The listing builds one solid part. Answer for the finished solid, in the listing's coordinates (mm). Face numbers are marked on the shaded views. A direction names the side the tool comes from. Coordinates: 2 decimals unless noted, no trailing zeros. Loops run counter-clockwise (first coordinate to the right, second up) from the corner with the lowest first, then second, coordinate; pieces in that order, holes last. Notation, with made-up numbers: M 55.5,58 L 91.5,58 A20 ccw 91.5,82 Z; hole C -5,-32 d1. An arc over 180 degrees is marked long. Answer as a JSON object with one key per item and string values. Group by question number.
1. A cutting plane is placed at B-B on x = 25.5. Give the vertices of the cut face in (y, z).
2. A cutting plane is placed at A-A on z = 12. Give the vertices of the cut face in (x, y) (3 decimals).
3. A cutting plane is placed at C-C on x = 12. Give the vertices of the cut face in (y, z), and give its area (3 significant figures).
4. Given pin 1 (4 mm diameter, centred on x = 14, z = 34, fed in from -Y); pin 2 (6 mm diameter, centred on x = -16.5, y = 81.5, fed in from -Z), each flat-ended and moving along its own axis, determine where each tip first touches the part or whether it passes through.
5. Determine the mould class of the marked faces 3, 4, 5 and 6 for opening direction X: released by +X, released by -X, zero draft, split by the parting line, or undercut.
6. For the marked faces 1 and 2, determine the directions among +Z, -Z, +X, -X, +Y, -Y from which every point of the face is accessible in a straight line to the end or side of a thin tool.
7. Straight lines are drawn through the part: L1, parallel to X at y = 76, z = 23.5; L2, parallel to Y at x = -11, z = 30; L3, parallel to Y at x = 19.5, z = 17.5. For each, find the intervals that lie inside material, in ascending order.
from build123d import *

# Parameters (mm, degrees)
BOSS_EXTRUDE1_DEPTH = 50.8
FILLET1_R           = 2.54


with BuildPart() as part:
    # Sketch1 → Boss-Extrude1 (new body)
    with BuildSketch(Plane.XY):
        with BuildLine():
            Line((-12.7, 73.846320157), (12.7, 73.846320157))
            Line((12.7, 73.846320157), (15.605843118, 90.742841512))
            ThreePointArc((15.605843118, 90.742841512), (23.776020133, 88.952270863), (31.75, 86.427675689))
            Line((31.75, 86.427675689), (31.75, 99.102275689))
            Line((31.75, 99.102275689), (-31.75, 99.102275689))
            Line((-31.75, 99.102275689), (-31.75, 86.427675689))
            ThreePointArc((-31.75, 86.427675689), (-23.776020133, 88.952270863), (-15.605843118, 90.742841512))
            Line((-15.605843118, 90.742841512), (-12.7, 73.846320157))
        make_face()
    extrude(amount=BOSS_EXTRUDE1_DEPTH)

    # Fillet1
    fillet1_edges = [part.edges().sort_by_distance(p)[0] for p in [
        (12.7, 73.846320157, 25.4),
        (-12.7, 73.846320157, 25.4),
        (-15.605843118, 90.742841512, 25.4),
        (15.605843118, 90.742841512, 25.4),
    ]]
    fillet(fillet1_edges, radius=FILLET1_R)


solid = part.part
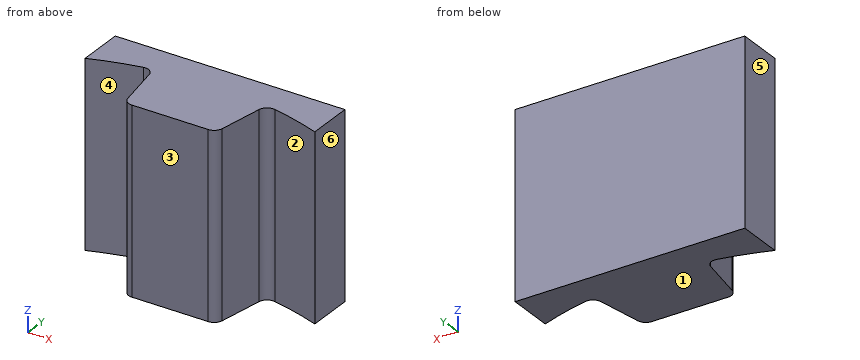
From the geometry:
{
 "1": {"outline": "M 88.47,0 L 99.1,0 L 99.1,50.8 L 88.47,50.8 Z"},
 "2": {"outline": "M -31.75,86.428 A92.075 cw -18.174,90.264 A2.54 cw -15.169,88.204 L -13.063,75.956 A2.54 ccw -10.56,73.846 L 10.56,73.846 A2.54 ccw 13.063,75.956 L 15.169,88.204 A2.54 cw 18.174,90.264 A92.075 cw 31.75,86.428 L 31.75,99.102 L -31.75,99.102 Z"},
 "3": {"outline": "M 74.29,0 L 99.1,0 L 99.1,50.8 L 74.29,50.8 Z", "area": "1,260 mm²"},
 "4": {"pin 1": "stops at y = 74.29", "pin 2": "stops at z = 0"},
 "5": {"face 3": "zero draft", "face 4": "undercut", "face 5": "released by -X", "face 6": "released by +X"},
 "6": {"face 1": "-Z, +X, -X, +Y, -Y", "face 2": "+Z, -Z, -Y"},
 "7": {"L1": "x = -13.07 to 13.07", "L2": "y = 73.88 to 99.1", "L3": "y = 89.99 to 99.1"}
}
